from build123d import *


with BuildPart() as part:
    # Sketch1 → Revolve1 (revolve)
    with BuildSketch(Plane(origin=(0, 0, 0), x_dir=(0, 0, -1), z_dir=(1, 0, 0))):
        with BuildLine():
            Line((1.190625, 4.7625), (1.5875, 4.7625))
            Line((1.5875, 4.7625), (1.5875, 4.206875))
            Line((1.5875, 4.206875), (1.5113, 4.206875))
            Line((1.5113, 4.206875), (1.5113, 3.730625))
            Line((1.5113, 3.730625), (0.1984375, 3.730625))
            Line((0.1984375, 3.730625), (0.1984375, 3.175))
            Line((0.1984375, 3.175), (1.5875, 3.175))
            Line((1.5875, 3.175), (1.5875, 2.69875))
            Line((1.5875, 2.69875), (1.5113, 2.69875))
            Line((1.5113, 2.69875), (1.5113, 2.06375))
            Line((1.5113, 2.06375), (1.5875, 2.06375))
            Line((1.5875, 2.06375), (1.5875, 1.5875))
            Line((1.5875, 1.5875), (-1.5875, 1.5875))
            Line((-1.5875, 1.5875), (-1.5875, 2.06375))
            Line((-1.5875, 2.06375), (-1.5113, 2.06375))
            Line((-1.5113, 2.06375), (-1.5113, 2.69875))
            Line((-1.5113, 2.69875), (-1.5875, 2.69875))
            Line((-1.5875, 2.69875), (-1.5875, 3.175))
            Line((-1.5875, 3.175), (-0.1984375, 3.175))
            Line((-0.1984375, 3.175), (-0.1984375, 3.730625))
            Line((-0.1984375, 3.730625), (-1.5113, 3.730625))
            Line((-1.5113, 3.730625), (-1.5113, 4.206875))
            Line((-1.5113, 4.206875), (-1.5875, 4.206875))
            Line((-1.5875, 4.206875), (-1.5875, 4.7625))
            Line((-1.5875, 4.7625), (-1.190625, 4.7625))
            Line((-1.190625, 4.7625), (-0.238125, 4.048125))
            ThreePointArc((-0.238125, 4.048125), (0, 3.96875), (0.238125, 4.048125))
            Line((0.238125, 4.048125), (1.190625, 4.7625))
        make_face()
    revolve(axis=Axis((0, 0, 1.5875), (0, 0, -1)))


solid = part.part
Geometry check sheet. Reference: the model listing, model coordinates, mm. A direction names the side the tool comes from. Coordinates: 2 decimals unless noted, no trailing zeros. Use one line per item in the form item = value. Start each with the question number.
Item 1: Gauge pin test, flat ends, axial feed: pin 1 (1.5 mm diameter, centred on x = 1.5, z = 0.5, fed in from +Y); pin 2 (1.5 mm diameter, centred on y = -0.5, z = 0, fed in from +X). Record the tip position at first contact, or that the pin passes through.
Item 2: Thickness scan on probe 1 along X at (y, z) = (0, -1.55) (1 decimal); probe 2 along Y at (x, z) = (-2.5, 1.45); probe 3 along Y at (x, z) = (2.5, -0.5). Record the ranges inside material, lowest first.
Item 3: Section check A-A, the plane z = -0.4. Give the number of separate pieces and of enclosed holes in the cut face, and give its area (3 significant figures).
Item 4: Mould release check, pull along X, two halves, no side actions. Record for faces 4 (the face through (-4, 0, -1.511)), 5 (the face through (-4, -2, 1.588)), 6 (the face through (-2.9, -3.78, -1.39)): +X half, -X half, draft (parallel to the pull), parting line (faces both ways), or undercut.
Item 5: Tool access check on faces 1 (the face through (-4, 0, 1.511)), 2 (the face through (-2, -1, -1.511)), 3 (the face through (-1.55, -0.34, 0.02)). Record the directions out of +Z, -Z, +X, -X, +Y, -Y that give a thin tool (end or side, any length) a straight path to the whole face; none if there is none.
Computed:
q1.pin_1 = 4.61
q1.pin_2 = 4.41
q2.probe_1 = -4.8 to -4.2, -3.2 to -2.7, -2.1 to -1.6, 1.6 to 2.1, 2.7 to 3.2, 4.2 to 4.8
q2.probe_2 = -4.05 to -2.77, -1.96 to 1.96, 2.77 to 4.05
q2.probe_3 = -3.43 to -2.77, -1.96 to 1.96, 2.77 to 3.43
q3.separate_pieces = 2
q3.enclosed_holes = 2
q3.area = 34.6 mm2
q4.face_4 = undercut
q4.face_5 = draft
q4.face_6 = parting line
q5.face_1 = +Z
q5.face_2 = -Z
q5.face_3 = +Z, -Z
